from build123d import *

# Parameters (mm, degrees)
CROQUIS1_R              = 1.85
SALIENTE_EXTRUIR1_DEPTH = 2.5
REDONDEO1_R             = 1


with BuildPart() as part:
    # Croquis1 → Saliente-Extruir1 (new body)
    with BuildSketch(Plane.XY):
        Polygon((-7.8, -16.5), (-5.65, -16.5), (0, -16.5), (5.65, -16.5), (7.8, -16.5), (7.8, -11.1), (5.65, -11.1), (5.65, 16.5), (-5.65, 16.5), (-5.65, -11.1), (-7.8, -11.1), align=None)
        with BuildLine():
            ThreePointArc((1.744493193, -8.435965803), (0, -10.180458996), (-1.744493193, -8.435965803))
            Line((-1.744493193, -8.435965803), (-1.744493193, -4.893383092))
            ThreePointArc((-1.744493193, -4.893383092), (0, -3.148889899), (1.744493193, -4.893383092))
            Line((1.744493193, -4.893383092), (1.744493193, -8.435965803))
        make_face(mode=Mode.SUBTRACT)
        with Locations((0, 11.5)):
            Circle(CROQUIS1_R, mode=Mode.SUBTRACT)
    extrude(amount=SALIENTE_EXTRUIR1_DEPTH)

    # Redondeo1
    redondeo1_edges = [part.edges().sort_by_distance(p)[0] for p in [
        (7.8, -11.1, 1.25),
        (7.8, -16.5, 1.25),
        (-7.8, -16.5, 1.25),
        (-7.8, -11.1, 1.25),
        (-5.65, 16.5, 1.25),
        (5.65, 16.5, 1.25),
    ]]
    fillet(redondeo1_edges, radius=REDONDEO1_R)


solid = part.part
The listing builds one solid part. Answer for the finished solid, in the listing's coordinates (mm). A direction names the side the tool comes from. Coordinates: 2 decimals unless noted, no trailing zeros. Loops run counter-clockwise (first coordinate to the right, second up) from the corner with the lowest first, then second, coordinate; pieces in that order, holes last. Notation, with made-up numbers: (-21.5, 26) -> (-15.5, 26) arc R20 cw to (-15.5, 51) -> close; hole circle Ø5 at (32, -16.75). An arc over 180 degrees is marked (long way). Answer in a Markdown table with one row per item. Add a question column.
1. The part is cut by section D-D, the plane y = 11.5. Write down the section's boundary in (x, z).
2. The part is cut by section B-B, the plane z = 1.4. Write down the section's boundary in (x, y).
3. Flat-ended cylindrical pins translate along their axes: P1, Ø0.8, axis at y = -7.5, z = 1, coming from the -X side; P2, Ø0.6, axis at x = -6, z = 1.5, coming from the +Y side; P3, Ø1, axis at y = 2, z = 0.5, coming from the +X side. Find the tip coordinate at first contact, or state that the pin passes through.
4. The part is cut by section C-C, the plane x = 0. Write down the section's boundary in (y, z).
5. The part is cut by section A-A, the plane y = -8. Write down the section's boundary in (x, z).
6. For faces 1 (the flat face through (0, 0, 2.5)), 2 (the flat face through (-7.8, -14, 1)), 3 (the flat face through (-6, -11.1, 1)), 4 (the cylindrical face through (-0.04, -3.15, 1.23)), 5 (the flat face through (6, -11.1, 1)), determine the directions among +Z, -Z, +X, -X, +Y, -Y from which every point of the face is accessible in a straight line to the end or side of a thin tool.
7. Consider line 1 (Y direction, x = 0, z = 0.55); line 2 (Y direction, x = 1, z = 0.65); line 3 (X direction, y = -7, z = 2.15). Determine where each line is inside the solid, lowest interval first. Write a range as [from, to].
Answer below:
| question | item | result |
|---|---|---|
| 1 | outline | (-5.65, 0) -> (-1.85, 0) -> (-1.85, 2.5) -> (-5.65, 2.5) -> close; (1.85, 0) -> (5.65, 0) -> (5.65, 2.5) -> (1.85, 2.5) -> close |
| 2 | outline | (-7.8, -15.5) arc R1 ccw to (-6.8, -16.5) -> (6.8, -16.5) arc R1 ccw to (7.8, -15.5) -> (7.8, -12.1) arc R1 ccw to (6.8, -11.1) -> (5.65, -11.1) -> (5.65, 15.5) arc R1 ccw to (4.65, 16.5) -> (-4.65, 16.5) arc R1 ccw to (-5.65, 15.5) -> (-5.65, -11.1) -> (-6.8, -11.1) arc R1 ccw to (-7.8, -12.1) -> close; hole circle Ø3.7 at (0, 11.5); hole (-1.74, -8.44) arc R1.74 ccw to (1.74, -8.44) -> (1.74, -4.89) arc R1.74 ccw to (-1.74, -4.89) -> close |
| 3 | P1 | x = -5.65 |
| 3 | P2 | y = -11.1 |
| 3 | P3 | x = 5.65 |
| 4 | outline | (-16.5, 0) -> (-10.18, 0) -> (-10.18, 2.5) -> (-16.5, 2.5) -> close; (-3.15, 0) -> (9.65, 0) -> (9.65, 2.5) -> (-3.15, 2.5) -> close; (13.35, 0) -> (16.5, 0) -> (16.5, 2.5) -> (13.35, 2.5) -> close |
| 5 | outline | (-5.65, 0) -> (-1.74, 0) -> (-1.74, 2.5) -> (-5.65, 2.5) -> close; (1.74, 0) -> (5.65, 0) -> (5.65, 2.5) -> (1.74, 2.5) -> close |
| 6 | face 1 | +Z, +X, -X, +Y, -Y |
| 6 | face 2 | +Z, -Z, -X, +Y, -Y |
| 6 | face 3 | +Z, -Z, -X, +Y |
| 6 | face 4 | +Z, -Z |
| 6 | face 5 | +Z, -Z, +X, +Y |
| 7 | line 1 | [-16.5, -10.18], [-3.15, 9.65], [13.35, 16.5] |
| 7 | line 2 | [-16.5, -9.87], [-3.46, 9.94], [13.06, 16.5] |
| 7 | line 3 | [-5.65, -1.74], [1.74, 5.65] |
